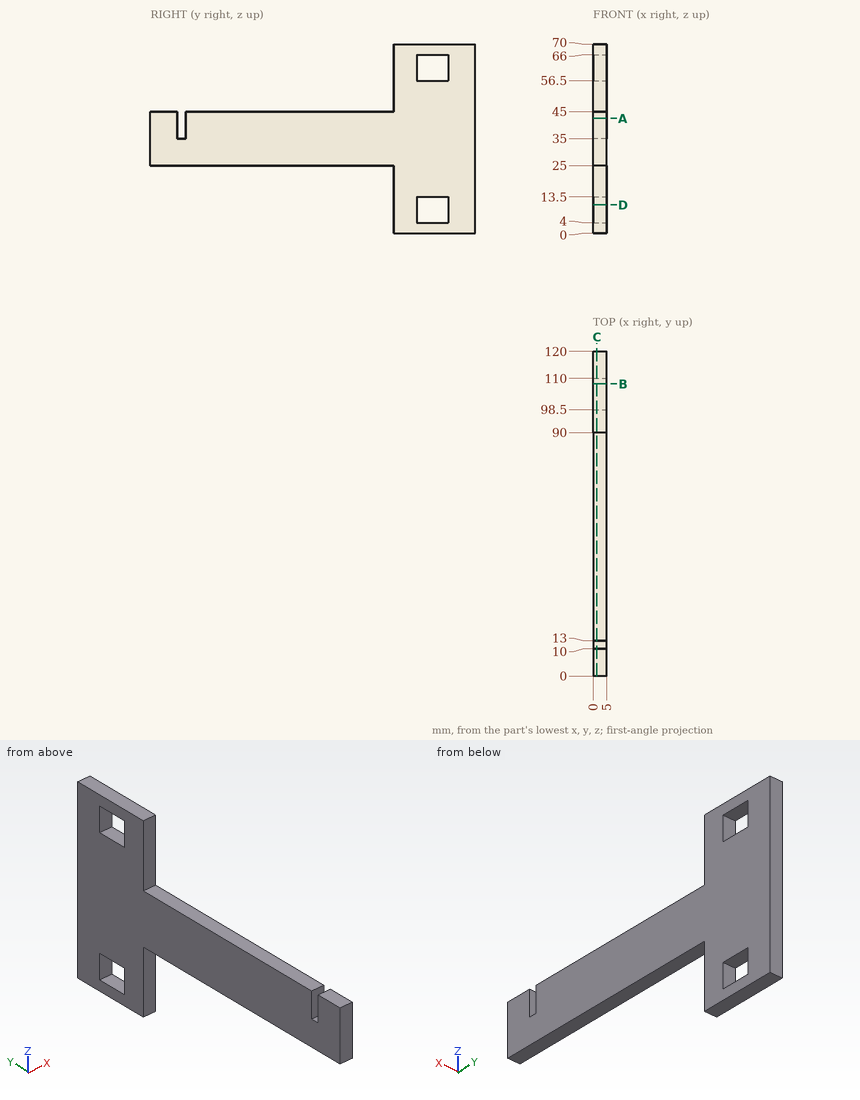
The drawing under review shows one solid part. Ordinate dimensions are in mm from its lowest x, y, z. Give positions to 0.01 mm unless a question says otherwise; leave off trailing zeros. Order: outer loops, then holes, each group sorted by start corner. A loop starts at its lowest first (then second) coordinate and runs counter-clockwise, first axis right, second up. Notation, with made-up numbers: M 78,-31 L 118,-31 A33 cw 118,6 Z; hole C 23,63.5 d5. An arc over 180 degrees is marked long. Answer in a Markdown table with one row per item. Add a question column.
1. To check wall thickness, follow line 1 along Z through (x, y) = (1.35, 100.5); line 2 along Y through (x, z) = (3, 43); line 3 along Y through (x, z) = (0.5, 17). State the ranges of each line that lie inside material, in increasing order.
2. For pin 1 Ø1.5 at (x, y) = (2, 33.5) entering from +Z; pin 2 Ø5 at (y, z) = (85, 21) entering from +X; pin 3 Ø1.5 at (x, y) = (3.5, 107) entering from -Z; pin 4 Ø1.5 at (x, z) = (2, 61.5) entering from -Y, all flat-tipped, find the tip position at first contact; note any pin that passes through.
3. Add section B-B on y = 108. State the section outline as (x, z) points.
4. Add section D-D on z = 10.5. State the section outline as (x, y) points, plus the area to 3 significant figures.
5. Add section C-C on x = 1.4. State the section outline as (y, z) points, plus the area to 3 significant figures.
6. Add section A-A on z = 42.5. State the section outline as (x, y) points, plus the area to 3 significant figures.
The answers:
| question | item | result |
|---|---|---|
| 1 | line 1 | 0 to 4, 13.5 to 56.5, 66 to 70 |
| 1 | line 2 | 0 to 10, 13 to 120 |
| 1 | line 3 | 90 to 120 |
| 2 | pin 1 | z = 45 |
| 2 | pin 2 | through |
| 2 | pin 3 | z = 0 |
| 2 | pin 4 | y = 90 |
| 3 | outline | M 0,0 L 5,0 L 5,4 L 0,4 Z; M 0,13.5 L 5,13.5 L 5,56.5 L 0,56.5 Z; M 0,66 L 5,66 L 5,70 L 0,70 Z |
| 4 | outline | M 0,90 L 5,90 L 5,98.5 L 0,98.5 Z; M 0,110 L 5,110 L 5,120 L 0,120 Z |
| 4 | area | 92.5 mm2 |
| 5 | outline | M 0,25 L 90,25 L 90,0 L 120,0 L 120,70 L 90,70 L 90,45 L 13,45 L 13,35 L 10,35 L 10,45 L 0,45 Z; hole M 98.5,4 L 110,4 L 110,13.5 L 98.5,13.5 Z; hole M 98.5,56.5 L 110,56.5 L 110,66 L 98.5,66 Z |
| 5 | area | 3,650 mm2 |
| 6 | outline | M 0,0 L 5,0 L 5,10 L 0,10 Z; M 0,13 L 5,13 L 5,120 L 0,120 Z |
| 6 | area | 585 mm2 |
